```python
from build123d import *

# Parameters (mm, degrees)
SKETCH2_W                                 = 40
SKETCH2_H                                 = 28
BOSS_EXTRUDE2_DEPTH                       = 50
SKETCH3_W                                 = 8
SKETCH3_H                                 = 28
BOSS_EXTRUDE3_DEPTH                       = 30
F_9_32_0_28125_DIAMETER_HOLE1_D           = 7.14375
F_9_32_0_28125_DIAMETER_HOLE1_CSINK_D     = 8.41375
F_9_32_0_28125_DIAMETER_HOLE1_CSINK_ANGLE = 90
FILLET5_R                                 = 15
FILLET3_R                                 = 15
FILLET4_R                                 = 15
FILLET6_R                                 = 15
FILLET7_R                                 = 3
FILLET8_R                                 = 3


with BuildPart() as part:
    # Sketch2 → Boss-Extrude2 (new body)
    with BuildSketch(Plane(origin=(0, 0, 0), x_dir=(1, 0, 0), z_dir=(0, 1, 0))):
        with Locations((20, 14)):
            Rectangle(SKETCH2_W, SKETCH2_H)
    extrude(amount=BOSS_EXTRUDE2_DEPTH)

    # Sketch3 → Boss-Extrude3 (add)
    with BuildSketch(Plane(origin=(0, 50, 0), x_dir=(1, 0, 0), z_dir=(0, 1, 0))):
        with Locations((4, 14)):
            Rectangle(SKETCH3_W, SKETCH3_H)
        with Locations((24.5, 14)):
            Rectangle(SKETCH3_W, SKETCH3_H)
    extrude(amount=BOSS_EXTRUDE3_DEPTH)

    # 9/32 (0.28125) Diameter Hole1 (through all)
    with Locations(Plane(origin=(0, 65, -12.5), x_dir=(0, 0, -1), z_dir=(-1, 0, 0))):
        with Locations((0, 0)):
            CounterSinkHole(F_9_32_0_28125_DIAMETER_HOLE1_D / 2, F_9_32_0_28125_DIAMETER_HOLE1_CSINK_D / 2, counter_sink_angle=F_9_32_0_28125_DIAMETER_HOLE1_CSINK_ANGLE)

    # Fillet5
    fillet5_edges = [part.edges().sort_by_distance(p)[0] for p in [
        (4, 80, 0),
    ]]
    fillet(fillet5_edges, radius=FILLET5_R)

    # Fillet3
    fillet3_edges = [part.edges().sort_by_distance(p)[0] for p in [
        (24.5, 80, -28),
    ]]
    fillet(fillet3_edges, radius=FILLET3_R)

    # Fillet4
    # the kernel refuses this fillet: 15 mm, written as the material it takes off along each edge
    with BuildSketch(Plane(origin=(65.665171868, 80, 0), x_dir=(0, 0, -1), z_dir=(-1, 0, 0))) as fillet4_piece_1:
        with BuildLine():
            CenterArc((15, 14.866068747), FILLET4_R, 180, 82.337744339)
            Line((0, 14.866068747), (-0.3, 14.866068747))
            Line((-0.3, 14.866068747), (-0.3, 0))
            Line((-0.3, 0), (0, -0.3))
            ThreePointArc((0, -0.3), (6.5, -0.3), (12.96, -0.297321375))
            Line((12.96, -0.297321375), (13, 0))
        make_face()
    extrude(amount=82.330343737, mode=Mode.SUBTRACT)

    # Fillet6
    # the kernel refuses this fillet: 15 mm, written as the material it takes off along each edge
    with BuildSketch(Plane(origin=(-37.165171868, 80, -28), x_dir=(0, -1, 0), z_dir=(1, 0, 0))) as fillet6_piece_1:
        with BuildLine():
            CenterArc((14.866068747, -15), FILLET6_R, 90, 82.337744339)
            Line((0, -13), (-0.297321375, -12.96))
            ThreePointArc((-0.297321375, -12.96), (-0.3, -6.5), (-0.3, 0))
            Line((-0.3, 0), (0, 0.3))
            Line((0, 0.3), (14.866068747, 0.3))
            Line((14.866068747, 0.3), (14.866068747, 0))
        make_face()
    extrude(amount=82.330343737, mode=Mode.SUBTRACT)

    # Fillet7
    # the kernel refuses this fillet: 3 mm, written as the material it takes off along each edge
    with BuildSketch(Plane(origin=(0, 65, 0), x_dir=(1, 0, 0), z_dir=(0, -1, 0))) as fillet7_piece_1:
        with BuildLine():
            CenterArc((FILLET7_R, -FILLET7_R), FILLET7_R, 90, 90)
            Line((0, -FILLET7_R), (0, 0))
            Line((0, 0), (FILLET7_R, 0))
        make_face()
    extrude(amount=72.5, mode=Mode.SUBTRACT)
    with BuildSketch(Plane(origin=(0, 65, -15), x_dir=(0, 0, 1), z_dir=(0, -1, 0))) as fillet7_piece_2:
        with BuildLine():
            CenterArc((15 - FILLET7_R, -FILLET7_R), FILLET7_R, 0, 90)
            Line((15, -FILLET7_R), (15, 0))
            Line((15, 0), (15 - FILLET7_R, 0))
        make_face()
    revolve(axis=Axis((0, 65, -15), (-1, 0, 0)), revolution_arc=118.659397847, mode=Mode.SUBTRACT)
    with BuildSketch(Plane(origin=(0, 65.133931253, -28), x_dir=(1, 0, 0), z_dir=(0, -1, 0))) as fillet7_piece_3:
        with BuildLine():
            CenterArc((FILLET7_R, FILLET7_R), FILLET7_R, 180, 90)
            Line((0, FILLET7_R), (0, 0))
            Line((0, 0), (FILLET7_R, 0))
        make_face()
    extrude(amount=72.633931253, mode=Mode.SUBTRACT)
    with BuildSketch(Plane(origin=(0, 65.133931253, -13), x_dir=(0, 0.933610035263845, 0.3582908065449657), z_dir=(0, -0.3582908065449657, 0.933610035263845))) as fillet7_piece_4:
        with BuildLine():
            CenterArc((15 - FILLET7_R, -FILLET7_R), FILLET7_R, 360, 90)
            Line((15, -FILLET7_R), (15, 0))
            Line((15, 0), (15 - FILLET7_R, 0))
        make_face()
    revolve(axis=Axis((0, 65.133931253, -13), (-1, 0, 0)), revolution_arc=110.995265648, mode=Mode.SUBTRACT)

    # Fillet8
    fillet8_edges = [part.edges().sort_by_distance(p)[0] for p in [
        (40, 25, -28),
        (40, 25, 0),
    ]]
    fillet(fillet8_edges, radius=FILLET8_R)


solid = part.part
```
Design review of the part built by this model. Coordinates are the model's own, in mm. A direction names the side the tool comes from. Coordinates: 2 decimals unless noted, no trailing zeros. Loops run counter-clockwise (first coordinate to the right, second up) from the corner with the lowest first, then second, coordinate; pieces in that order, holes last. Notation, with made-up numbers: (63.5, -31.75) -> (109.5, -31.75) arc R15 ccw to (109.5, -9.75) -> close; hole circle Ø9 at (81, 71). An arc over 180 degrees is marked (long way). Answer as a JSON object with one key per item and string values.
Q1. Take a section at C-C on x = 32.5. Give the boundary of the cut face in (y, z), plus the area to 3 significant figures.
Answer block:
{"outline": "(0, -28) -> (50, -28) -> (50, 0) -> (0, 0) -> close", "area": "1,400 mm^2"}
Q2. Take a section at B-B on x = 27.5. Give the boundary of the cut face in (y, z).
Answer block:
{"outline": "(0, -28) -> (65, -28) arc R15 ccw to (80, -13) arc R15 ccw to (65.13, 0) -> (0, 0) -> close; hole circle Ø7.14 at (65, -12.5)"}
Q3. The part is to be moulded in two halves that separate along X. For faces 1 (the cylindrical face through (0.86, 33.02, -27.1)), 2 (the flat face through (8, 61, -14)), 3 (the cylindrical face through (39.1, 25.35, -27.14)), 4 (the flat face through (34, 50, -14)), say which applies: +X half, -X half, draft (parallel to the pull), parting line (faces both ways), or undercut.
Answer block:
{"face 1": "-X half", "face 2": "undercut", "face 3": "+X half", "face 4": "draft"}
Q4. Clearance check with flat-ended pins moving along their axes: pin 1 Ø3 at (y, z) = (56, -12) entering from +X; pin 2 Ø1.5 at (x, z) = (12, -11.5) entering from +Y. State where each tip first meets the part, or that it passes through.
Answer block:
{"pin 1": "stops at x = 28.5", "pin 2": "stops at y = 50"}
Q5. Tool access review of faces 5 (the cylindrical face through (24.56, 75.49, -23.72)), 6 (the flat face through (14, 50, -14)), 7 (the flat face through (28.5, 61, -14)), 8 (the cylindrical face through (24.556, 61.459, -12.965)): name each direction out of +Z, -Z, +X, -X, +Y, -Y from which nothing blocks a thin tool from reaching the whole face with its end or side.
Answer block:
{"face 5": "-Z, +X, +Y", "face 6": "+Z, -Z, +Y", "face 7": "+Z, -Z, +X, +Y", "face 8": "+X, -X"}
Q6. To check wall thickness, follow L1, parallel to Z at x = 22.5, y = 65; L2, parallel to X at y = 59.5, z = -7.75; L3, parallel to Y at x = 18.5, z = -19. State the ranges of each line that lie inside material, in increasing order.
Answer block:
{"L1": "z = -28 to -16.07, -8.93 to 0", "L2": "x = 0 to 8, 20.5 to 28.5", "L3": "y = 0 to 50"}
Q7. Take a section at A-A on y = 53. Give the boundary of the cut face in (x, z), plus the area to 3 significant figures.
Answer block:
{"outline": "(0, -25) arc R3 ccw to (3, -28) -> (8, -28) -> (8, 0) -> (3, 0) arc R3 ccw to (0, -3) -> close; (20.5, -28) -> (28.5, -28) -> (28.5, 0) -> (20.5, 0) -> close", "area": "444 mm^2"}
